from build123d import *

# Parameters (mm, degrees)
F0_R     = 76.2
F0_R_2   = 50.8
F1_DEPTH = 2.54
F3_DEPTH = 25.4


with BuildPart() as f1:
    # F0 (on Front) → F1 (new body)
    with BuildSketch(Plane.XZ):
        Circle(F0_R)
        Circle(F0_R_2, mode=Mode.SUBTRACT)
    extrude(amount=F1_DEPTH)

    # F2 (on face) → F3 (cut)
    with BuildSketch(Plane.XZ.offset(2.54)):
        Polygon((-6.221704, 77.47), (0, 69.85), (6.221704, 77.47), align=None)
    extrude(amount=-F3_DEPTH, mode=Mode.SUBTRACT)


solid = f1.part
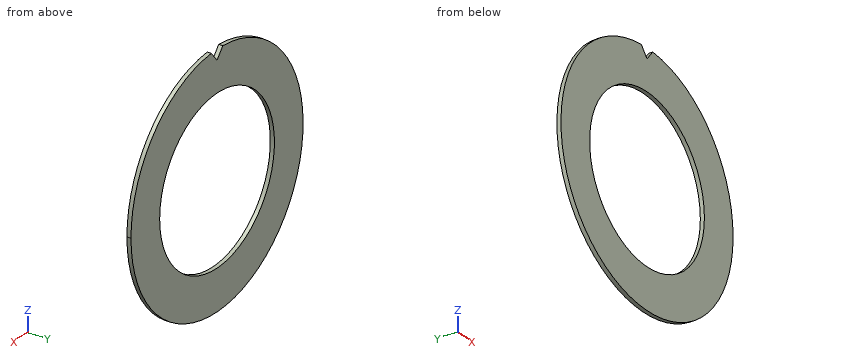
For this review, take the finished solid that the model builds, in its own axes (mm). Round coordinates to 2 decimals unless told otherwise and drop trailing zeros. Loops run counter-clockwise (first coordinate to the right, second up) from the corner with the lowest first, then second, coordinate; pieces in that order, holes last. Notation, with made-up numbers: (-23.5, -34) - (6.5, -34) arc R22 cw to (6.5, -9) - close; hole circle Ø6 at (-2, 68). An arc over 180 degrees is marked (long way). Use one line per item in the form item = value.
Item 1: Consider section D-D on z = 66. Write out the cut boundary in (x, y).
Answers:
outline = (-38.08, -2.54) - (38.08, -2.54) - (38.08, 0) - (-38.08, 0) - close
Item 2: Clearance check with flat-ended pins moving along their axes: P1, Ø5, axis at x = -0.5, z = -46, coming from the -Y side; P2, Ø1, axis at x = 26, y = -0.5, coming from the +Z side; P3, Ø12, axis at x = 28.5, z = -57.5, coming from the +Y side; P4, Ø1.5, axis at x = -55.5, y = -0.5, coming from the +Z side. State where each tip first meets the part, or that it passes through.
Answers:
P1 = through
P2 = 71.81
P3 = 0
P4 = 53
Item 3: For line 1 (Z direction, x = 0, y = -0.6); line 2 (X direction, y = -1.45, z = 2.5); line 3 (X direction, y = -0.7, z = -7.5), list the stretches that pass through material, from the lowest coordinate up.
Answers:
line_1 = -76.2 to -50.8, 50.8 to 69.85
line_2 = -76.16 to -50.74, 50.74 to 76.16
line_3 = -75.83 to -50.24, 50.24 to 75.83
Item 4: Consider section A-A on x = -44. Write out the cut boundary in (y, z).
Answers:
outline = (-2.54, -62.21) - (0, -62.21) - (0, -25.39) - (-2.54, -25.39) - close; (-2.54, 25.39) - (0, 25.39) - (0, 62.21) - (-2.54, 62.21) - close
Item 5: Consider section C-C on y = -1.9. Write out the cut boundary in (x, z).
Answers:
outline = (-5.05, 76.03) arc R76.2 ccw (long way) to (5.05, 76.03) - (0, 69.85) - close; hole circle Ø101.6 at (0, 0)
Item 6: Consider section B-B on z = 3. Write out the cut boundary in (x, y), then the cut area to 3 significant figures.
Answers:
outline = (-76.14, -2.54) - (-50.71, -2.54) - (-50.71, 0) - (-76.14, 0) - close; (50.71, -2.54) - (76.14, -2.54) - (76.14, 0) - (50.71, 0) - close
area = 129 mm^2
